Verification items for the finished model (mm, model axes). Coordinates: 2 decimals unless noted, no trailing zeros. Write each loop counter-clockwise with the first axis right and the second up, starting at its lowest first coordinate (ties: lowest second). Pieces come first, ordered by that corner, then holes. Notation, with made-up numbers: (67, -10) -> (100, -10) arc R20 cw to (100, 7) -> close; hole circle Ø6 at (52, 2). An arc over 180 degrees is marked (long way). Use CSV: the item, a comma, the result in double quotes.
```python
from build123d import *

# Parameters (mm, degrees)
SKETCH_1_R             = 13.5
SM_BASE_FLANGE_1_DEPTH = 4


# Sheet-metal steps are written as plain solids
with BuildPart() as part:
    # Sketch 1 → Базовая кромка1 (new body)
    with BuildSketch(Plane.XY):
        with BuildLine():
            Line((0, -35), (250, -35))
            Line((250, -35), (250, 6.5))
            Line((250, 6.5), (50, 6.5))
            ThreePointArc((50, 6.5), (38.424329978, 27.637073819), (39.947947324, 51.688074136))
            ThreePointArc((39.947947324, 51.688074136), (39.067621468, 56.60193476), (34.375031444, 58.305049172))
            Line((34.375031444, 58.305049172), (-35, 46.072359341))
            Line((-35, 46.072359341), (-35, -35))
            Line((-35, -35), (0, -35))
        make_face()
        Circle(SKETCH_1_R, mode=Mode.SUBTRACT)
    extrude(amount=-SM_BASE_FLANGE_1_DEPTH)


solid = part.part
```
1) Scan lines: L1, parallel to Y at x = 0, z = -2.45; L2, parallel to Y at x = -7.5, z = -0.35; L3, parallel to X at y = -9, z = -1.4. Record each from-to range of solid material in increasing order.
Return value:
L1,"-35 to -13.5, 13.5 to 52.24"
L2,"-35 to -11.22, 11.22 to 50.92"
L3,"-35 to -10.06, 10.06 to 250"
2) Cross-section at A-A (y = 0). Record the boundary of the cut face in (x, z), plus the area to 3 significant figures.
Return value:
outline,"(-35, -4) -> (-13.5, -4) -> (-13.5, 0) -> (-35, 0) -> close; (13.5, -4) -> (250, -4) -> (250, 0) -> (13.5, 0) -> close"
area,"1,030 mm2"
3) Cross-section at B-B (z = -3.1). Record the boundary of the cut face in (x, y).
Return value:
outline,"(-35, -35) -> (250, -35) -> (250, 6.5) -> (50, 6.5) arc R43.28 cw to (39.95, 51.69) arc R5 ccw to (34.38, 58.31) -> (-35, 46.07) -> close; hole circle Ø27 at (0, 0)"
4) Gauge pin test, flat end, axial feed: pin 1 (1.5 mm diameter, centred on x = 199, z = -1, fed in from +Y). Record the tip position at first contact, or that the pin passes through.
Return value:
pin 1,"y = 6.5"
5) Cross-section at D-D (x = 95.5). Record the boundary of the cut face in (y, z), plus the area to 3 significant figures.
Return value:
outline,"(-35, -4) -> (6.5, -4) -> (6.5, 0) -> (-35, 0) -> close"
area,"166 mm2"
6) Cross-section at C-C (x = 0). Record the boundary of the cut face in (y, z).
Return value:
outline,"(-35, -4) -> (-13.5, -4) -> (-13.5, 0) -> (-35, 0) -> close; (13.5, -4) -> (52.24, -4) -> (52.24, 0) -> (13.5, 0) -> close"
7) Mould release check, pull along Y, two halves, no side actions. Record for faces 1 (the cylindrical face through (-2.93, -13.18, -1.97)), 2 (the cylindrical face through (38.5, 27.3, -2)), 3 (the flat face through (0.173, 52.274, -1.972)), 4 (the flat face through (74, -8, -4)): released by +Y, released by -Y, zero draft, split by the parting line, or undercut.
Return value:
face 1,"undercut"
face 2,"undercut"
face 3,"released by +Y"
face 4,"zero draft"
